Can you work these out from the model? Positions are in its coordinate system, mm. Give positions to 0.01 mm unless a question says otherwise; leave off trailing zeros. Write each loop counter-clockwise with the first axis right and the second up, starting at its lowest first coordinate (ties: lowest second). Pieces come first, ordered by that corner, then holes.
1. If I drill on probe 1 along Y at (x, z) = (13.5, 8); probe 2 along Z at (x, y) = (1, 5.5); probe 3 along Z at (x, y) = (8.25, -7), over which ranges is the centre line in solid material (lowest first)?
2. Suppose I cut it at C-C (y = 9.5). Please give me the cut outline in (x, z).
3. Suppose I cut it at A-A (z = 0). Please give me the cut outline in (x, y), and give its area (3 significant figures).
4. Suppose I cut it at D-D (y = -4.25). Please give me the cut outline in (x, z).
5. Suppose I cut it at B-B (z = 7). Please give me the cut outline in (x, y).
6. I'm going to push flat-ended pins straight in: pin 1 (6 mm diameter, centred on x = 6, y = -3.5, fed in from +Z); pin 2 (1.3 mm diameter, centred on x = 6, z = 0, fed in from -Y); pin 3 (1 mm diameter, centred on x = 3.5, z = 7.5, fed in from -Y). Where does each tip first touch, or does it pass through?
7. Thinking about a two-plate mould opening in Z: for faces 1 (the flat face through (15, -5, 0)), 2 (the cylindrical face through (7.4, -6.06, 4.42)), 3 (the cylindrical face through (7.4, 2.92, 2.93)), which applies, pulls with the +Z half, pulls with the -Z half, needs draft (parallel to the pull), parting line crosses it, or undercut?
```python
from build123d import *

# Parameters (mm, degrees)
SPUR_GEAR_GB_BORE_OUTLINE_R = 1
SPUR_GEAR_GB_BORE_DEPTH     = 15
CUT_EXTRUDE_3_DEPTH         = 15


# Read off the part's stored shape, not the designer's step: <spur gear_gb>-<Bore>
with BuildPart() as part:
    # <spur gear_gb>-<Bore> outline → <spur gear_gb>-<Bore> (new body)
    with BuildSketch(Plane.YZ):
        with BuildLine():
            ThreePointArc((-0.256880001, -11.997250213), (0, -12), (0.256880001, -11.997250213))
            ThreePointArc((0.256880001, -11.997250213), (1.456299749, -9.849931218), (1.172541409, -7.406763642))
            ThreePointArc((1.172541409, -7.406763642), (2.317318441, -7.131972816), (3.404980509, -6.681400207))
            ThreePointArc((3.404980509, -6.681400207), (4.61147306, -8.824753264), (6.843986457, -9.856969584))
            ThreePointArc((6.843986457, -9.856969584), (7.053423027, -9.708203933), (7.259627029, -9.554989032))
            ThreePointArc((7.259627029, -9.554989032), (6.967815552, -7.112770233), (5.302192362, -5.302995112))
            ThreePointArc((5.302192362, -5.302995112), (6.066818441, -4.407801607), (6.681915604, -3.403968986))
            ThreePointArc((6.681915604, -3.403968986), (8.917819898, -4.428819506), (11.330682707, -3.9516616))
            ThreePointArc((11.330682707, -3.9516616), (11.412678196, -3.708203933), (11.489443278, -3.463046803))
            ThreePointArc((11.489443278, -3.463046803), (9.817862641, -1.658772773), (7.406586048, -1.173662691))
            ThreePointArc((7.406586048, -1.173662691), (7.499, 0), (7.406586048, 1.173662691))
            ThreePointArc((7.406586048, 1.173662691), (9.817862641, 1.658772773), (11.489443278, 3.463046803))
            ThreePointArc((11.489443278, 3.463046803), (11.412678196, 3.708203933), (11.330682707, 3.9516616))
            ThreePointArc((11.330682707, 3.9516616), (8.917819898, 4.428819506), (6.681915604, 3.403968986))
            ThreePointArc((6.681915604, 3.403968986), (6.066818441, 4.407801607), (5.302192362, 5.302995112))
            ThreePointArc((5.302192362, 5.302995112), (6.967815552, 7.112770233), (7.259627029, 9.554989032))
            ThreePointArc((7.259627029, 9.554989032), (7.053423027, 9.708203933), (6.843986457, 9.856969584))
            ThreePointArc((6.843986457, 9.856969584), (4.61147306, 8.824753264), (3.404980509, 6.681400207))
            ThreePointArc((3.404980509, 6.681400207), (2.317318441, 7.131972816), (1.172541409, 7.406763642))
            ThreePointArc((1.172541409, 7.406763642), (1.456299749, 9.849931218), (0.256880001, 11.997250213))
            ThreePointArc((0.256880001, 11.997250213), (0, 12), (-0.256880001, 11.997250213))
            ThreePointArc((-0.256880001, 11.997250213), (-1.456299749, 9.849931218), (-1.172541409, 7.406763642))
            ThreePointArc((-1.172541409, 7.406763642), (-2.317318441, 7.131972816), (-3.404980509, 6.681400207))
            ThreePointArc((-3.404980509, 6.681400207), (-4.61147306, 8.824753264), (-6.843986457, 9.856969584))
            ThreePointArc((-6.843986457, 9.856969584), (-7.053423027, 9.708203933), (-7.259627029, 9.554989032))
            ThreePointArc((-7.259627029, 9.554989032), (-6.967815552, 7.112770233), (-5.302192362, 5.302995112))
            ThreePointArc((-5.302192362, 5.302995112), (-6.066818441, 4.407801607), (-6.681915604, 3.403968986))
            ThreePointArc((-6.681915604, 3.403968986), (-8.917819898, 4.428819506), (-11.330682707, 3.9516616))
            ThreePointArc((-11.330682707, 3.9516616), (-11.412678196, 3.708203933), (-11.489443278, 3.463046803))
            ThreePointArc((-11.489443278, 3.463046803), (-9.817862641, 1.658772773), (-7.406586048, 1.173662691))
            ThreePointArc((-7.406586048, 1.173662691), (-7.499, 0), (-7.406586048, -1.173662691))
            ThreePointArc((-7.406586048, -1.173662691), (-9.817862641, -1.658772773), (-11.489443278, -3.463046803))
            ThreePointArc((-11.489443278, -3.463046803), (-11.412678196, -3.708203933), (-11.330682707, -3.9516616))
            ThreePointArc((-11.330682707, -3.9516616), (-8.917819898, -4.428819506), (-6.681915604, -3.403968986))
            ThreePointArc((-6.681915604, -3.403968986), (-6.066818441, -4.407801607), (-5.302192362, -5.302995112))
            ThreePointArc((-5.302192362, -5.302995112), (-6.967815552, -7.112770233), (-7.259627029, -9.554989032))
            ThreePointArc((-7.259627029, -9.554989032), (-7.053423027, -9.708203933), (-6.843986457, -9.856969584))
            ThreePointArc((-6.843986457, -9.856969584), (-4.61147306, -8.824753264), (-3.404980509, -6.681400207))
            ThreePointArc((-3.404980509, -6.681400207), (-2.317318441, -7.131972816), (-1.172541409, -7.406763642))
            ThreePointArc((-1.172541409, -7.406763642), (-1.456299749, -9.849931218), (-0.256880001, -11.997250213))
        make_face()
        Circle(SPUR_GEAR_GB_BORE_OUTLINE_R, mode=Mode.SUBTRACT)
    extrude(amount=SPUR_GEAR_GB_BORE_DEPTH)

    # 草图8 → 切除-拉伸3 (cut)
    with BuildSketch(Plane(origin=(0, 0, 0), x_dir=(0, 0, -1), z_dir=(1, 0, 0))):
        with BuildLine():
            Line((-2.217335854, 3.217335854), (2.217335854, 3.217335854))
            ThreePointArc((2.217335854, 3.217335854), (2.924442636, 2.924442636), (3.217335854, 2.217335854))
            Line((3.217335854, 2.217335854), (3.217335854, -2.217335854))
            ThreePointArc((3.217335854, -2.217335854), (2.924442636, -2.924442636), (2.217335854, -3.217335854))
            Line((2.217335854, -3.217335854), (-2.217335854, -3.217335854))
            ThreePointArc((-2.217335854, -3.217335854), (-2.924442636, -2.924442636), (-3.217335854, -2.217335854))
            Line((-3.217335854, -2.217335854), (-3.217335854, 2.217335854))
            ThreePointArc((-3.217335854, 2.217335854), (-2.924442636, 2.924442636), (-2.217335854, 3.217335854))
        make_face()
    extrude(amount=CUT_EXTRUDE_3_DEPTH, mode=Mode.SUBTRACT)


solid = part.part
```
Checks:
1. probe 1: y = -7.26 to -3.93, -1.39 to 1.39, 3.93 to 7.26
1. probe 2: z = -9.45 to -5.42, -5.1 to 5.1, 5.42 to 9.45
1. probe 3: z = -9.75 to -7.18, -3.67 to 3.67, 7.18 to 9.75
2. outline: (0, -4.45) - (15, -4.45) - (15, -1.5) - (0, -1.5) - close; (0, 1.5) - (15, 1.5) - (15, 4.45) - (0, 4.45) - close
3. outline: (0, -7.5) - (15, -7.5) - (15, -3.22) - (0, -3.22) - close; (0, 3.22) - (15, 3.22) - (15, 7.5) - (0, 7.5) - close
3. area: 128 mm2
4. outline: (0, -8.44) - (15, -8.44) - (15, 8.44) - (0, 8.44) - close
5. outline: (0, -6.91) - (15, -6.91) - (15, -3.48) - (0, -3.48) - close; (0, -2.69) - (15, -2.69) - (15, 2.69) - (0, 2.69) - close; (0, 3.48) - (15, 3.48) - (15, 6.91) - (0, 6.91) - close
6. pin 1: stops at z = 11.75
6. pin 2: stops at y = -7.5
6. pin 3: stops at y = -7.26
7. face 1: needs draft
7. face 2: undercut
7. face 3: undercut
